```python
from build123d import *

# Parameters (mm, degrees)
F0_W     = 31.28
F0_H     = 27.35
F1_DEPTH = 11.1252
F2_W     = 3.4544
F2_H     = 9.0932
F2_W_2   = 3.7464
F2_H_2   = 9.0805
F3_DEPTH = 27.351


with BuildPart() as f1:
    # F0 (on Top) → F1 (new body)
    with BuildSketch(Plane.XY):
        with Locations((-15.64, 13.675)):
            Rectangle(F0_W, F0_H)
    extrude(amount=F1_DEPTH)

    # F2 (on face) → F3 (cut, through all)
    with BuildSketch(Plane.XZ):
        with Locations((-24.168, 6.5786)):
            Rectangle(F2_W, F2_H)
        with Locations((-19.977, 6.5786)):
            Rectangle(F2_W, F2_H)
        with Locations((-15.786, 6.5786)):
            Rectangle(F2_W, F2_H)
        with Locations((-11.595, 6.5786)):
            Rectangle(F2_W, F2_H)
        with Locations((-7.258, 6.5786)):
            Rectangle(F2_W_2, F2_H)
        with Locations((-2.921, 6.58495)):
            Rectangle(F2_W, F2_H_2)
        with Locations((-28.359, 6.58495)):
            Rectangle(F2_W, F2_H_2)
    extrude(amount=-F3_DEPTH, mode=Mode.SUBTRACT)


solid = f1.part
```
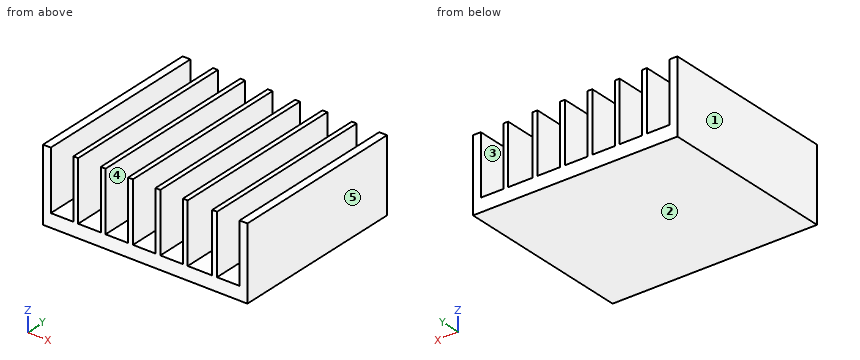
Input: part model. Units: mm. Frame: model coordinates. Face numbers are marked on the shaded views. A direction names the side the tool comes from. Give positions to 0.01 mm unless a question says otherwise; leave off trailing zeros. Order: outer loops, then holes, each group sorted by start corner. A loop starts at its lowest first (then second) coordinate and runs counter-clockwise, first axis right, second up. Notation, with made-up numbers: (23, -37.5) - (57, -37.5) arc R27 cw to (57, -8.5) - close; hole circle Ø1 at (25, 53). An arc over 180 degrees is marked (long way). Use a Markdown table: item, result.
(1) Section query D-D (x = -15.5). Output: boundary loops of the cut face in (y, z), then the cut area to 3 significant figures.
Computed values:
| item | result |
|---|---|
| outline | (0, 0) - (27.35, 0) - (27.35, 2.03) - (0, 2.03) - close |
| area | 55.6 mm2 |
(2) Line query: line 1 (Z direction, x = -30, y = 15.75). Output: solid intervals per line, ascending. Write a range as from..to.
Computed values:
| item | result |
|---|---|
| line 1 | z = 0..2.04 |
(3) Section query C-C (x = -28). Output: boundary loops of the cut face in (y, z).
Computed values:
| item | result |
|---|---|
| outline | (0, 0) - (27.35, 0) - (27.35, 2.04) - (0, 2.04) - close |
(4) Pin query (flat end, axial travel): pin 1 (1.9 mm diameter, centred on x = -7, y = 19.5, fed in from +Z). Return the tip coordinate at first contact, or that it passes through.
Computed values:
| item | result |
|---|---|
| pin 1 | stops at z = 2.03 |
(5) Access query for the marked faces 4 and 5. Directions: +Z, -Z, +X, -X, +Y, -Y. A direction counts if a zero-diameter tool reaches every point of the face in a straight line with its end or side. Return the directions, or none.
Computed values:
| item | result |
|---|---|
| face 4 | +Z, +Y, -Y |
| face 5 | +Z, -Z, +X, +Y, -Y |
(6) Section query A-A (z = 6.5). State how many separate pieces and enclosed holes the cut face has, then the cut area to 3 significant figures.
Computed values:
| item | result |
|---|---|
| separate pieces | 8 |
| enclosed holes | 0 |
| area | 186 mm2 |
(7) Draft query along X for the marked faces 1, 2 and 3. Return one class per face: released by +X, released by -X, zero draft, split by the parting line, or undercut.
Computed values:
| item | result |
|---|---|
| face 1 | released by -X |
| face 2 | zero draft |
| face 3 | undercut |
